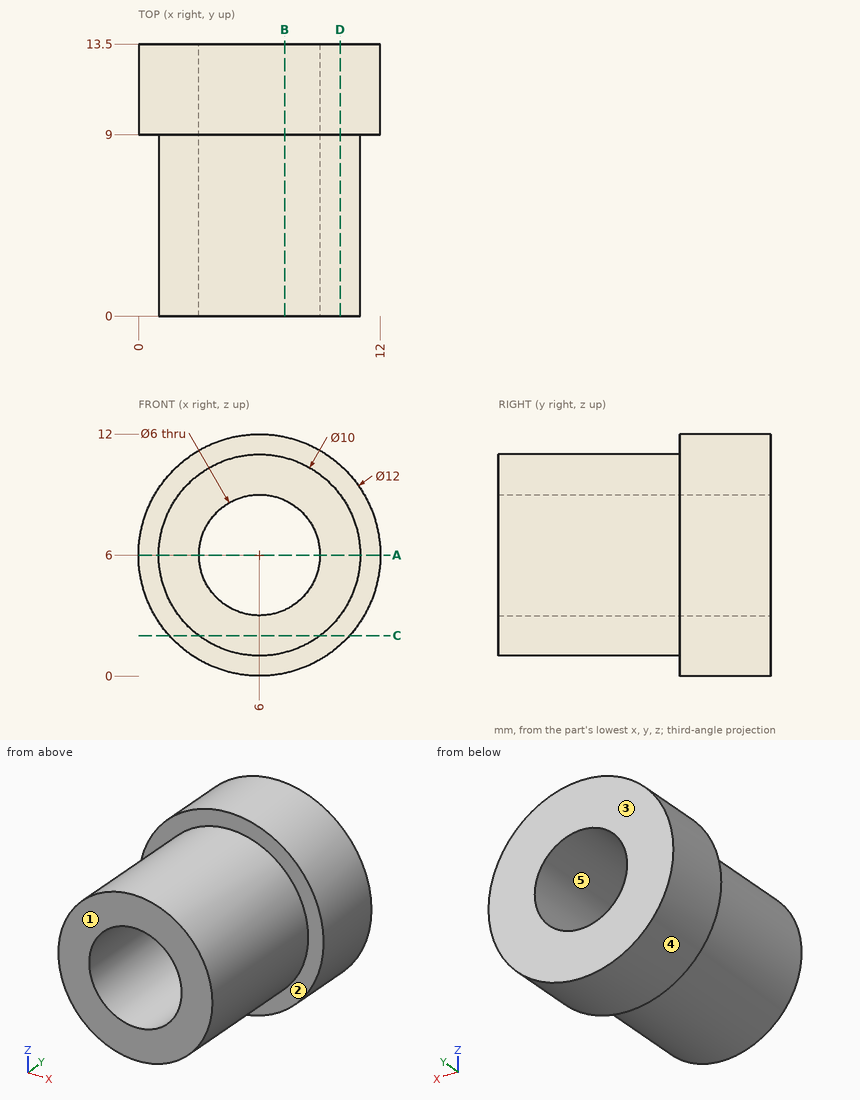
Could you check a few things on this drawing? It's one solid part, dimensions in mm from its lowest x, y, z. A direction names the side the tool comes from. Coordinates: 2 decimals unless noted, no trailing zeros. Write each loop counter-clockwise with the first axis right and the second up, starting at its lowest first coordinate (ties: lowest second). Pieces come first, ordered by that corner, then holes. Notation, with made-up numbers: (16, 31.5) - (50, 31.5) arc R37 cw to (50, 67.5) - close; hole circle Ø10 at (-20.5, 50.5). An arc over 180 degrees is marked (long way). Use one line per item in the form item = value.
1) Thinking about a two-plate mould opening in X: for the marked faces 3, 4 and 5, which applies, released by +X, released by -X, zero draft, split by the parting line, or undercut?
Solved:
face_3 = zero draft
face_4 = split by the parting line
face_5 = undercut
2) I'm going to push flat-ended pins straight in: P1, Ø3, axis at x = 4, y = 2, coming from the -Z side; P2, Ø3, axis at x = 3, y = 10, coming from the -Z side; P3, Ø3, axis at y = 7, z = 3, coming from the -X side. Where does each tip first touch, or does it pass through?
Solved:
P1 = 1.03
P2 = 0.19
P3 = 1.23
3) I need wall thicknesses on line 1 (X direction, y = 6.25, z = 6); line 2 (X direction, y = 9.5, z = 6). Which ranges of each line are inside material? Lowest first, please.
Solved:
line_1 = 1 to 3, 9 to 11
line_2 = 0 to 3, 9 to 12
4) On a 3-axis mill with a long thin cutter (end or side, diameter ignored), from which of +Z, -Z, +X, -X, +Y, -Y can I reach the whole of each face in a straight line? I mean the marked faces 1 and 2. Say none if no direction works.
Solved:
face_1 = +Z, -Z, +X, -X, -Y
face_2 = -Y
5) Suppose I cut it at B-B, the plane x = 7.25. Write out the boundary of the cut face in (y, z).
Solved:
outline = (0, 1.16) - (9, 1.16) - (9, 0.13) - (13.5, 0.13) - (13.5, 3.27) - (0, 3.27) - close; (0, 8.73) - (13.5, 8.73) - (13.5, 11.87) - (9, 11.87) - (9, 10.84) - (0, 10.84) - close
6) Suppose I cut it at C-C, the plane z = 2. Write out the boundary of the cut face in (x, y), plus the area to 3 significant figures.
Solved:
outline = (1.53, 9) - (3, 9) - (3, 0) - (9, 0) - (9, 9) - (10.47, 9) - (10.47, 13.5) - (1.53, 13.5) - close
area = 94.2 mm2
7) Suppose I cut it at D-D, the plane x = 10. Write out the boundary of the cut face in (y, z), plus the area to 3 significant figures.
Solved:
outline = (0, 3) - (9, 3) - (9, 1.53) - (13.5, 1.53) - (13.5, 10.47) - (9, 10.47) - (9, 9) - (0, 9) - close
area = 94.2 mm2
8) Suppose I cut it at A-A, the plane z = 6. Write out the boundary of the cut face in (x, y).
Solved:
outline = (0, 9) - (1, 9) - (1, 0) - (3, 0) - (3, 13.5) - (0, 13.5) - close; (9, 0) - (11, 0) - (11, 9) - (12, 9) - (12, 13.5) - (9, 13.5) - close
